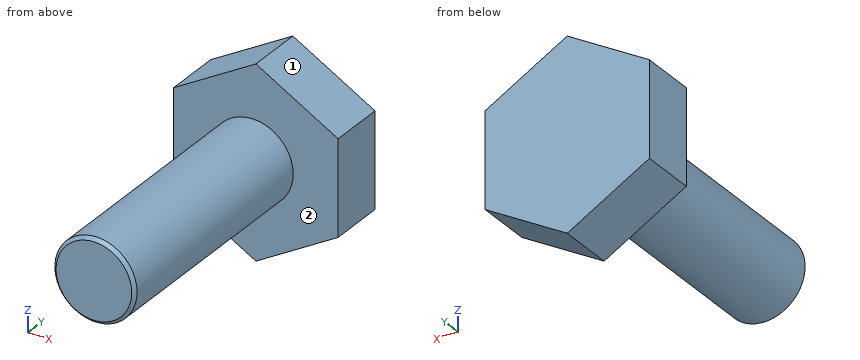
```python
from build123d import *

# Parameters (mm, degrees)
F1_DEPTH = 35
F2_R     = 25
F3_DEPTH = 150
F4_SIZE  = 2


with BuildPart() as f1:
    # F0 (on Front) → F1 (new body)
    with BuildSketch(Plane.XZ):
        Polygon((52.348992, -28.867513), (52.348992, 28.867513), (2.348992, 57.735027), (-47.651008, 28.867513), (-47.651008, -28.867513), (2.348992, -57.735027), align=None)
    extrude(amount=F1_DEPTH)

    # F2 (on face) → F3 (join)
    with BuildSketch(Plane.XZ.offset(35)):
        Circle(F2_R)
    extrude(amount=F3_DEPTH)

    # F4
    f4_edges = [f1.edges().sort_by_distance(p)[0] for p in [
        (-25, -185, 0),
    ]]
    chamfer(f4_edges, length=F4_SIZE)


solid = f1.part
```
For this review, take the finished solid that the model builds, in its own axes (mm). Face numbers are marked on the shaded views. A direction names the side the tool comes from. Round coordinates to 2 decimals unless told otherwise and drop trailing zeros. Write each loop counter-clockwise with the first axis right and the second up, starting at its lowest first coordinate (ties: lowest second). Pieces come first, ordered by that corner, then holes. Notation, with made-up numbers: (61.5, 58) -> (106.5, 58) arc R14 ccw to (106.5, 67) -> close; hole circle Ø11 at (-0.75, -40). An arc over 180 degrees is marked (long way). Use one line per item in the form item = value.
Q1. Consider section D-D (z = -50). State the section outline as (x, y) points.
Resolved:
outline = (-11.05, -35) -> (15.75, -35) -> (15.75, 0) -> (-11.05, 0) -> close
Q2. Consider section B-B (x = 0). State the section outline as (y, z) points.
Resolved:
outline = (-185, -23) -> (-183, -25) -> (-35, -25) -> (-35, -56.38) -> (0, -56.38) -> (0, 56.38) -> (-35, 56.38) -> (-35, 25) -> (-183, 25) -> (-185, 23) -> close
Q3. To check wall thickness, follow probe 1 along Y at (x, z) = (-29, -29.5); probe 2 along X at (y, z) = (-48.5, 14.5); probe 3 along Z at (x, y) = (-8, -167). State the ranges of each line that lie inside material, in increasing order. Write a range as from..to.
Resolved:
probe_1 = -35..0
probe_2 = -20.37..20.37
probe_3 = -23.69..23.69
Q4. Clearance check with flat-ended pins moving along their axes: pin 1 Ø2 at (y, z) = (-128.5, 22.5) entering from -X; pin 2 Ø8 at (y, z) = (-83.5, 22) entering from +X; pin 3 Ø5 at (x, z) = (30, -19.5) entering from -Y. State where each tip first meets the part, or that it passes through.
Resolved:
pin_1 = -12.76
pin_2 = 17.35
pin_3 = -35
Q5. Machinability: for the marked faces 1 and 2, which of the approach directions +Z, -Z, +X, -X, +Y, -Y give a long, thin tool a straight path to every point of the face, cutting with its end or side? Answer none if there is none.
Resolved:
face_1 = +Z, +X, +Y, -Y
face_2 = -Y
Q6. Consider section A-A (z = 0). State the section outline as (x, y) points.
Resolved:
outline = (-47.65, -35) -> (-25, -35) -> (-25, -183) -> (-23, -185) -> (23, -185) -> (25, -183) -> (25, -35) -> (52.35, -35) -> (52.35, 0) -> (-47.65, 0) -> close
Q7. Consider section C-C (y = -82). State the section outline as (x, z) points.
Resolved:
outline = circle Ø50 at (0, 0)
